Input: part model. Units: mm. Frame: model coordinates. A direction names the side the tool comes from. Round coordinates to 2 decimals unless told otherwise and drop trailing zeros. Write each loop counter-clockwise with the first axis right and the second up, starting at its lowest first coordinate (ties: lowest second). Pieces come first, ordered by that corner, then holes. Notation, with made-up numbers: M 22.5,82 L 65.5,82 A8 cw 65.5,96 Z; hole C 46.25,28.5 d8. An arc over 180 degrees is marked long. Answer as CSV lines item,"result". Start each with the question number.
```python
from build123d import *

# Parameters (mm, degrees)
BOSS_EXTRUDE1_DEPTH = 10
BOSS_EXTRUDE2_DEPTH = 3
FILLET1_R           = 1
FILLET2_R           = 1
FILLET3_R           = 1
FILLET4_R           = 1


with BuildPart() as part:
    # Sketch1 → Boss-Extrude1 (new body)
    with BuildSketch(Plane(origin=(0, 0, 0), x_dir=(1, 0, 0), z_dir=(0, 1, 0))):
        with BuildLine():
            ThreePointArc((4.75, -8.227241336), (0, -9.5), (-4.75, -8.227241336))
            Line((-4.75, -8.227241336), (-3.375, -5.845671476))
            ThreePointArc((-3.375, -5.845671476), (0, -6.75), (3.375, -5.845671476))
            Line((3.375, -5.845671476), (4.75, -8.227241336))
        make_face()
    extrude(amount=BOSS_EXTRUDE1_DEPTH)

    # Sketch2 → Boss-Extrude2 (add)
    with BuildSketch(Plane(origin=(0, 10, 0), x_dir=(1, 0, 0), z_dir=(0, 1, 0))):
        with BuildLine():
            Line((-3.375, -5.845671476), (-3.375, -15.845671476))
            Line((-3.375, -15.845671476), (3.375, -15.845671476))
            Line((3.375, -15.845671476), (3.375, -5.845671476))
            ThreePointArc((3.375, -5.845671476), (0, -6.75), (-3.375, -5.845671476))
        make_face()
    extrude(amount=BOSS_EXTRUDE2_DEPTH)

    # Fillet1
    fillet1_edges = [part.edges().sort_by_distance(p)[0] for p in [
        (0, 10, 9.5),
    ]]
    fillet(fillet1_edges, radius=FILLET1_R)

    # Fillet2
    fillet2_edges = [part.edges().sort_by_distance(p)[0] for p in [
        (-4.075600712, 10, 8.581344815),
    ]]
    fillet(fillet2_edges, radius=FILLET2_R)

    # Fillet3
    # the kernel refuses this fillet: 1 mm, written as the material it takes off along each edge
    with BuildSketch(Plane(origin=(-4.75, -2.798981274, 8.227241336), x_dir=(0.893983522608317, 0, 0.44809983408256804), z_dir=(0, 1, 0))) as fillet3_piece_1:
        with BuildLine():
            CenterArc((1.060666588, 0.998262358), FILLET3_R, 176.621836485, 96.756327031)
            Line((0.06240423, 1.05718828), (0, 0))
            ThreePointArc((0, 0), (0.559796255, -0.016507597), (1.11959251, 0))
        make_face()
    extrude(amount=14.597962548, mode=Mode.SUBTRACT)
    with BuildSketch(Plane(origin=(0, 10, 0), x_dir=(0.7080675160533174, 0, 0.706144739207257), z_dir=(0.706144739207257, 0, -0.7080675160533174))) as fillet3_piece_2_section:
        with BuildLine():
            CenterArc((9.5 - FILLET3_R, FILLET3_R), FILLET3_R, 270, 90)
            Line((9.5 - FILLET3_R, 0), (9.5, 0))
            Line((9.5, 0), (9.5, FILLET3_R))
        make_face()
    fillet3_piece_2 = revolve(axis=Axis((0, 10, 0), (0, -1, 0)), revolution_arc=39.346226133, mode=Mode.PRIVATE)
    fillet3_piece_2 = split(fillet3_piece_2, bisect_by=Plane(origin=(3.375, 9.768637129, 8.366507066), z_dir=(1, 0, 0)), keep=Keep.TOP, mode=Mode.PRIVATE)
    add(fillet3_piece_2, mode=Mode.SUBTRACT)

    # Fillet4
    # the kernel refuses this fillet: 1 mm, written as the material it takes off along each edge
    with BuildSketch(Plane(origin=(4.75, -2.798981274, 8.227241336), x_dir=(-0.8939835226083171, 0, 0.44809983408256765), z_dir=(0, 1, 0))) as fillet4_piece_1:
        with BuildLine():
            CenterArc((1.060666588, -0.998262358), FILLET4_R, 86.621836485, 96.756327031)
            Line((0.06240423, -1.05718828), (0, 0))
            ThreePointArc((0, 0), (0.559796255, 0.016507597), (1.11959251, 0))
        make_face()
    extrude(amount=14.597962548, mode=Mode.SUBTRACT)


solid = part.part
```
Item 1: Draft query along Y for faces 4 (the face through (0, 10, 13)), 5 (the face through (3.6, 10, 7)), 6 (the face through (-4.31, 4.93, 8.11)). Return one class per face: +Y half, -Y half, draft (parallel to the pull), parting line (faces both ways), or undercut.
Item 2: Access query for faces 1 (the face through (0.05, 6.41, 6.75)), 2 (the face through (0.1, 4.4, 9.5)), 3 (the face through (-3.6, 10, 7)). Directions: +Z, -Z, +X, -X, +Y, -Y. A direction counts if a zero-diameter tool reaches every point of the face in a straight line with its end or side. Return the directions, or none.
Item 3: Cut plane D-D, the plane z = 15.25. Return loops of the section in (x, y) (3 decimals), plus the area to 4 significant figures.
Item 4: Pin query (flat end, axial travel): pin 1 Ø5 at (y, z) = (10.5, 14) entering from -X (3 decimals); pin 2 Ø2 at (y, z) = (11, 8.5) entering from +X (3 decimals); pin 3 Ø4 at (y, z) = (4, 10.5) entering from +X; pin 4 Ø1 at (y, z) = (2, 10.5) entering from -X. Return the tip coordinate at first contact, or that it passes through.
Item 5: Cut plane C-C, the plane y = 8.75. Return loops of the section in (x, z) (3 decimals).
Item 6: Cut plane A-A, the plane z = 6.5. Return loops of the section in (x, y) (3 decimals).
Item 7: Cut plane B-B, the plane x = 0. Return loops of the section in (y, z).
Item 8: Line query: line 1 (Y direction, x = -3.25, z = 10.5); line 2 (Y direction, x = 4, z = 7); line 3 (Z direction, x = 0, y = 2.25). Output: solid intervals per line, ascending. Write a range as [from, to].
Results list:
1,face 4,"-Y half"
1,face 5,"+Y half"
1,face 6,"draft"
2,face 1,"-Z, +Y, -Y"
2,face 2,"+Z, -Y"
2,face 3,"+Z, -Z, -X, +Y"
3,outline,"M -3.375,10 L 3.375,10 L 3.375,13 L -3.375,13 Z"
3,area,"20.25 mm²"
4,pin 1,"x = -3.375"
4,pin 2,"x = 3.375"
4,pin 3,"x = 4.08"
4,pin 4,"through"
5,outline,"M -4.22,7.31 L -3.375,5.846 A6.75 cw 3.375,5.846 L 4.22,7.31 A1 ccw 3.749,8.729 A9.5 ccw -3.749,8.729 A1 ccw Z"
6,outline,"M -3.753,0 L -1.82,0 L -1.82,13 L -3.375,13 L -3.375,10 L -3.753,10 Z; M 1.82,0 L 3.753,0 L 3.753,10 L 3.375,10 L 3.375,13 L 1.82,13 Z"
7,outline,"M 0,6.75 L 13,6.75 L 13,15.85 L 10,15.85 L 10,10.5 A1 cw 9,9.5 L 0,9.5 Z"
8,line 1,"[10, 13]"
8,line 2,"[0, 10]"
8,line 3,"[6.75, 9.5]"
